For this review, take the finished solid that the model builds, in its own axes (mm). A direction names the side the tool comes from. Round coordinates to 2 decimals unless told otherwise and drop trailing zeros. Write each loop counter-clockwise with the first axis right and the second up, starting at its lowest first coordinate (ties: lowest second). Pieces come first, ordered by that corner, then holes. Notation, with made-up numbers: M 62,64.25 L 101,64.25 A13 cw 101,88.25 Z; hole C 59,50.25 d5. An arc over 180 degrees is marked long. Use one line per item in the form item = value. Start each with the question number.
Item 1: Add section C-C (z = 106.5). State the section outline as (x, y) points.
Item 2: Add section B-B (y = 10). State the section outline as (x, z) points, and give its area (3 significant figures).
Item 3: For P1, Ø7, axis at x = -1151.5, y = 38, coming from the -Z side; P2, Ø4, axis at x = -1462, y = -6, coming from the -Z side; P3, Ø1.5, axis at x = -1232, y = 10.5, coming from the -Z side, all flat-tipped, find the tip position at first contact; note any pin that passes through.
Item 4: Add section A-A (x = -474.5). State the section outline as (y, z) points, and give its area (3 significant figures).
Item 5: For line 1 (Z direction, x = -912, y = -23); line 2 (Z direction, x = -1393, y = 40.5); line 3 (X direction, y = -8.5, z = 774.5), list the stretches that pass through material, from the lowest coordinate up. Write a range as [from, to].
Item 6: For faces 3 (the flat face through (-314.56, 37.44, 186.16)), 4 (the flat face through (-1471.45, 39.08, 855.44)), list the 3-axis set-ups (+Z, -Z, +X, -X, +Y, -Y) from which the entire face can be reached by the end or side of a thin tool; tool diameter is ignored.
Item 7: Add section D-D (x = -1404). Count the separate pieces of the cut face and the enclosed holes in it, and give its area (3 significant figures).
Item 8: Draft analysis for pull direction Z (two halves, no side actions). For faces 1 (the flat face through (-887.4, -0.63, 410.176)), 2 (the flat face through (-620, 42, 1080)), state which applies: released by +Z, released by -Z, zero draft, split by the parting line, or undercut.
from build123d import *

# Parameters (mm, degrees)
F6_W     = 90
F6_H     = 203.898897171
F7_DEPTH = 1800.001


with BuildPart() as f2:
    # F2: sweep along a path in F0
    with BuildLine(Plane.XZ) as f2_path:
        Line((0, 0), (0, 1100))
        Line((0, 1100), (-1800, 1100))
        Line((-1800, 1100), (-1800, 832))
        Line((-1800, 832), (0, 0))
    # F1 (on Top) → F2 (sweep)
    with BuildSketch(Plane.XY):
        Polygon((0, -45), (0, 0), (0, 45), (-40, 45), (-40, 33), (-37, 33), (-37, 42), (-3, 42), (-3, 0), (-3, -42), (-37, -42), (-37, -33), (-40, -33), (-40, -45), align=None)
    sweep(path=f2_path.line, transition=Transition.RIGHT)

    # F5: sweep along a path in F3
    with BuildLine(Plane.XZ) as f5_path:
        Line((-600, 1100), (-600, 277.3333333333))
        Line((-600, 277.3333333333), (-1200, 1100))
        Line((-1200, 1100), (-1200, 554.6666666667))
        Line((-1200, 554.6666666667), (-1800, 1100))
    # F4 (on face) → F5 (sweep)
    with BuildSketch(Plane.XY.offset(1100)):
        Polygon((-600, -45), (-600, 0), (-600, 45), (-640, 45), (-640, 33), (-637, 33), (-637, 42), (-603, 42), (-603, 0), (-603, -42), (-637, -42), (-637, -33), (-640, -33), (-640, -45), align=None)
    sweep(path=f5_path.line, transition=Transition.RIGHT)

    # F6 (on face) → F7 (cut, through all)
    with BuildSketch(Plane.YZ):
        with Locations((0, 1201.9494485855)):
            Rectangle(F6_W, F6_H)
    extrude(amount=-F7_DEPTH, mode=Mode.SUBTRACT)


solid = f2.part
Calculated:
q1.outline = M -230.41,-45 L -135.07,-45 L -135.07,-33 L -142.22,-33 L -142.22,-42 L -223.26,-42 L -223.26,42 L -142.22,42 L -142.22,33 L -135.07,33 L -135.07,45 L -230.41,45 Z; M -40,-45 L 0,-45 L 0,45 L -40,45 L -40,33 L -37,33 L -37,42 L -3,42 L -3,-42 L -37,-42 L -37,-33 L -40,-33 Z
q2.outline = M -1800,832 L 0,0 L 0,1100 L -1800,1100 Z; hole M -1797,833.92 L -1207.4,561.39 L -1796.7,1097 L -1797,1097 Z; hole M -1792.24,1097 L -1203,561.45 L -1203,1097 Z; hole M -1200,557.97 L -603.64,282.32 L -1197.81,1097 L -1200,1097 Z; hole M -1194.1,1097 L -603,286.54 L -603,1097 Z; hole M -600,280.64 L -3,4.69 L -3,1097 L -600,1097 Z
q2.area = 24,900 mm^2
q3.P1 = 530.63
q3.P2 = 674.84
q3.P3 = 569.11
q4.outline = M -45,219.32 L 45,219.32 L 45,263.39 L 33,263.39 L 33,260.09 L 42,260.09 L 42,222.63 L -42,222.63 L -42,260.09 L -33,260.09 L -33,263.39 L -45,263.39 Z; M -45,1060 L -33,1060 L -33,1063 L -42,1063 L -42,1097 L 42,1097 L 42,1063 L 33,1063 L 33,1060 L 45,1060 L 45,1100 L -45,1100 Z
q4.area = 1,150 mm^2
q5.line_1 = [421.55, 424.85], [705.12, 710.21], [1097, 1100]
q5.line_2 = [643.88, 647.18], [684.64, 687.94], [730.08, 734.14], [780.08, 784.14], [1060, 1063], [1097, 1100]
q5.line_3 = [-1675.6, -1668.45], [-1441.87, -1437.41], [-1203, -1200], [-962.6, -958.89], [-603, -600], [-3, 0]
q6.face_3 = none
q6.face_4 = +Y, -Y
q7.separate_pieces = 3
q7.enclosed_holes = 0
q7.area = 1,890 mm^2
q8.face_1 = released by -Z
q8.face_2 = undercut
